```python
from build123d import *

# Parameters (mm, degrees)
SALIENTE_EXTRUIR1_DEPTH = 30
CROQUIS2_R              = 9
CORTAR_EXTRUIR1_DEPTH   = 110.733009315
CROQUIS3_R              = 9
CORTAR_EXTRUIR2_DEPTH   = 30
CROQUIS4_R              = 9
CORTAR_EXTRUIR3_DEPTH   = 30


with BuildPart() as part:
    # Croquis1 → Saliente-Extruir1 (new body)
    with BuildSketch(Plane.XY):
        Polygon((-20, 0), (20, 0), (20, 20), (96, -23.878620458), (96, -43.878620458), (94.2, -43.878620458), (94.2, -24.917850943), (21.8, 16.882308546), (21.8, -1.8), (-21.8, -1.8), (-21.8, 16.882308546), (-94.2, -24.917850943), (-94.2, -43.878620458), (-96, -43.878620458), (-96, -23.878620458), (-20, 20), align=None)
    extrude(amount=SALIENTE_EXTRUIR1_DEPTH)

    # Croquis2 → Cortar-Extruir1 (cut, through all)
    with BuildSketch(Plane(origin=(0, 0, 0), x_dir=(1, 0, 0), z_dir=(0, 1, 0))):
        with Locations(Location((0, -15, 0), (0, 0, 180))):
            Circle(CROQUIS2_R)
    extrude(amount=-CORTAR_EXTRUIR1_DEPTH, mode=Mode.SUBTRACT)

    # Croquis3 → Cortar-Extruir2 (cut)
    with BuildSketch(Plane(origin=(13.660254038, 23.660254038, 0), x_dir=(0.866025403784438, -0.5000000000000012, 0), z_dir=(0.5000000000000012, 0.866025403784438, 0))):
        with Locations(Location((51.199128534, -15, 0), (0, 0, 180))):
            Circle(CROQUIS3_R)
    extrude(amount=-CORTAR_EXTRUIR2_DEPTH, mode=Mode.SUBTRACT)

    # Croquis4 → Cortar-Extruir3 (cut)
    with BuildSketch(Plane(origin=(-13.660254038, 23.660254038, 0), x_dir=(0.8660254037844378, 0.5000000000000017, 0), z_dir=(-0.5000000000000016, 0.8660254037844377, 0))):
        with Locations(Location((-51.199128534, -15, 0), (0, 0, 180))):
            Circle(CROQUIS4_R)
    extrude(amount=-CORTAR_EXTRUIR3_DEPTH, mode=Mode.SUBTRACT)


solid = part.part
```
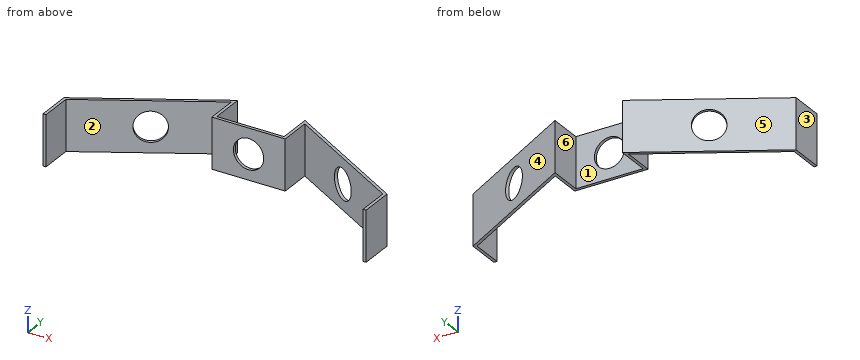
CAD build for the part. Positions are in the model's coordinates, mm. Face numbers are marked on the shaded views. A direction names the side the tool comes from. Give positions to 0.01 mm unless a question says otherwise; leave off trailing zeros. Write each loop counter-clockwise with the first axis right and the second up, starting at its lowest first coordinate (ties: lowest second). Pieces come first, ordered by that corner, then holes. Notation, with made-up numbers: M 48,24.25 L 85,24.25 A14 cw 85,40.25 Z; hole C 66,54 d11. An arc over 180 degrees is marked long. Return JSON: item names as keys, results as strings. Group by question number.
(1) Band-saw the part on D-D (x = -78.5). Give the cut face in (y, z) (3 decimals).
(2) Mould opens along X. For the marked faces 4, 5 and 6 say: pulls with the +X half, pulls with the -X half, needs draft (parallel to the pull), parting line crosses it, or undercut.
(3) Band-saw the part on B-B (x = 0). Give the cut face in (y, z), and give its area (3 significant figures).
(4) Flat gauge pins, fed straight in: pin 1 Ø5 at (x, z) = (21, 11.5) entering from -Y; pin 2 Ø6 at (y, z) = (10, 13) entering from -X; pin 3 Ø1.5 at (y, z) = (5, 25) entering from +X; pin 4 Ø11 at (x, z) = (0, 15) entering from +Y. Where does each tip first touch, or does it go through?
(5) Drill centre lines: L1, parallel to Z at x = 0, y = -0.4; L2, parallel to X at y = 10, z = 3.5; L3, parallel to X at y = -41, z = 4. Where is each one in solid material? Low to high. Write a range as [from, to].
(6) Band-saw the part on C-C (z = 15). Give the cut face in (x, y), and give its area (3 significant figures).
(7) Band-saw the part on A-A (y = -38). Give the cut face in (x, z), and give its area (3 significant figures).
(8) 3-axis set-ups, long thin cutter, end or side, ignore diameter. For the marked faces 1, 2 and 3: which of +Z, -Z, +X, -X, +Y, -Y reach the whole face in a straight line?
Entries:
{
 "1": {"outline": "M -15.853,0 L -13.775,0 L -13.775,30 L -15.853,30 Z"},
 "2": {"face 4": "pulls with the +X half", "face 5": "pulls with the -X half", "face 6": "undercut"},
 "3": {"outline": "M -1.8,0 L 0,0 L 0,6 L -1.8,6 Z; M -1.8,24 L 0,24 L 0,30 L -1.8,30 Z", "area": "21.6 mm^2"},
 "4": {"pin 1": "stops at y = -1.8", "pin 2": "stops at x = -42.52", "pin 3": "stops at x = 47.28", "pin 4": "passes through"},
 "5": {"L1": "z = [0, 6], [24, 30]", "L2": "x = [-37.32, -33.72], [-21.8, -20], [20, 21.8], [33.72, 37.32]", "L3": "x = [-96, -94.2], [94.2, 96]"},
 "6": {"outline": "M -96,-43.88 L -94.2,-43.88 L -94.2,-24.92 L -64.89,-8 L -65.79,-6.44 L -96,-23.88 Z; M -50.21,2.56 L -49.31,1 L -21.8,16.88 L -21.8,-1.8 L -9,-1.8 L -9,0 L -20,0 L -20,20 Z; M 9,-1.8 L 21.8,-1.8 L 21.8,16.88 L 49.31,1 L 50.21,2.56 L 20,20 L 20,0 L 9,0 Z; M 64.89,-8 L 94.2,-24.92 L 94.2,-43.88 L 96,-43.88 L 96,-23.88 L 65.79,-6.44 Z", "area": "426 mm^2"},
 "7": {"outline": "M -96,0 L -94.2,0 L -94.2,30 L -96,30 Z; M 94.2,0 L 96,0 L 96,30 L 94.2,30 Z", "area": "108 mm^2"},
 "8": {"face 1": "+Z, -Z, +Y", "face 2": "+Z, -Z, -Y", "face 3": "+Z, -Z, -X, +Y, -Y"}
}
